from build123d import *

# Parameters (mm, degrees)
SKETCH_1_W      = 3
SKETCH_1_H      = 20
SKETCH_1_W_2    = 20
SKETCH_1_H_2    = 3
EXTRUDE_1_DEPTH = 6
FILLET_2_R      = 15
FILLET_3_R      = 15
FILLET_4_R      = 15
FILLET_5_R      = 15
FILLET_6_R      = 15
FILLET_7_R      = 15
FILLET_8_R      = 15
FILLET_9_R      = 15
FILLET_10_R     = 15
FILLET_11_R     = 15
FILLET_12_R     = 15
FILLET_13_R     = 15
FILLET_14_R     = 15
FILLET_15_R     = 15


with BuildPart() as part:
    # Эскиз1 → Бобышка-Вытянуть1 (new body)
    with BuildSketch(Plane.XY):
        Polygon((118, 244), (118, 129), (268, 129), (268, 244), (293, 244), (293, 250), (313, 250), (313, 244), (356, 244), (356, 250), (376, 250), (376, 244), (386, 244), (386, 147), (392, 147), (392, 97), (386, 97), (386, 0), (366, 0), (366, -6), (346, -6), (346, 0), (203, 0), (203, -6), (183, -6), (183, 0), (40, 0), (40, -6), (20, -6), (20, 0), (0, 0), (0, 97), (-6, 97), (-6, 147), (0, 147), (0, 244), (10, 244), (10, 250), (30, 250), (30, 244), (73, 244), (73, 250), (93, 250), (93, 244), align=None)
        Polygon((20, 20), (20, 224), (88, 224), (88, 99), (183, 99), (183, 20), align=None, mode=Mode.SUBTRACT)
        Polygon((298, 99), (298, 224), (366, 224), (366, 20), (203, 20), (203, 99), align=None, mode=Mode.SUBTRACT)
        with Locations((99.5, 214)):
            Rectangle(SKETCH_1_W, SKETCH_1_H, mode=Mode.SUBTRACT)
        with Locations((99.5, 159)):
            Rectangle(SKETCH_1_W, SKETCH_1_H, mode=Mode.SUBTRACT)
        with Locations((148, 110.5)):
            Rectangle(SKETCH_1_W_2, SKETCH_1_H_2, mode=Mode.SUBTRACT)
        with Locations((238, 110.5)):
            Rectangle(SKETCH_1_W_2, SKETCH_1_H_2, mode=Mode.SUBTRACT)
        with Locations((286.5, 214)):
            Rectangle(SKETCH_1_W, SKETCH_1_H, mode=Mode.SUBTRACT)
        with Locations((286.5, 159)):
            Rectangle(SKETCH_1_W, SKETCH_1_H, mode=Mode.SUBTRACT)
    extrude(amount=EXTRUDE_1_DEPTH)

    # Скругление2
    fillet_2_edges = [part.edges().sort_by_distance(p)[0] for p in [
        (366, 20, 3),
    ]]
    fillet(fillet_2_edges, radius=FILLET_2_R)

    # Скругление3
    fillet_3_edges = [part.edges().sort_by_distance(p)[0] for p in [
        (203, 99, 3),
    ]]
    fillet(fillet_3_edges, radius=FILLET_3_R)

    # Скругление4
    fillet_4_edges = [part.edges().sort_by_distance(p)[0] for p in [
        (203, 20, 3),
    ]]
    fillet(fillet_4_edges, radius=FILLET_4_R)

    # Скругление5
    fillet_5_edges = [part.edges().sort_by_distance(p)[0] for p in [
        (298, 99, 3),
    ]]
    fillet(fillet_5_edges, radius=FILLET_5_R)

    # Скругление6
    fillet_6_edges = [part.edges().sort_by_distance(p)[0] for p in [
        (298, 224, 3),
    ]]
    fillet(fillet_6_edges, radius=FILLET_6_R)

    # Скругление7
    fillet_7_edges = [part.edges().sort_by_distance(p)[0] for p in [
        (366, 224, 3),
    ]]
    fillet(fillet_7_edges, radius=FILLET_7_R)

    # Скругление8
    fillet_8_edges = [part.edges().sort_by_distance(p)[0] for p in [
        (183, 99, 3),
    ]]
    fillet(fillet_8_edges, radius=FILLET_8_R)

    # Скругление9
    fillet_9_edges = [part.edges().sort_by_distance(p)[0] for p in [
        (20, 224, 3),
    ]]
    fillet(fillet_9_edges, radius=FILLET_9_R)

    # Скругление10
    fillet_10_edges = [part.edges().sort_by_distance(p)[0] for p in [
        (88, 99, 3),
    ]]
    fillet(fillet_10_edges, radius=FILLET_10_R)

    # Скругление11
    fillet_11_edges = [part.edges().sort_by_distance(p)[0] for p in [
        (88, 224, 3),
    ]]
    fillet(fillet_11_edges, radius=FILLET_11_R)

    # Скругление12
    fillet_12_edges = [part.edges().sort_by_distance(p)[0] for p in [
        (183, 20, 3),
    ]]
    fillet(fillet_12_edges, radius=FILLET_12_R)

    # Скругление13
    fillet_13_edges = [part.edges().sort_by_distance(p)[0] for p in [
        (20, 20, 3),
    ]]
    fillet(fillet_13_edges, radius=FILLET_13_R)

    # Скругление14
    fillet_14_edges = [part.edges().sort_by_distance(p)[0] for p in [
        (268, 129, 3),
    ]]
    fillet(fillet_14_edges, radius=FILLET_14_R)

    # Скругление15
    fillet_15_edges = [part.edges().sort_by_distance(p)[0] for p in [
        (118, 129, 3),
    ]]
    fillet(fillet_15_edges, radius=FILLET_15_R)


solid = part.part
For this review, take the finished solid that the model builds, in its own axes (mm). A direction names the side the tool comes from. Round coordinates to 2 decimals unless told otherwise and drop trailing zeros. Order: outer loops, then holes, each group sorted by start corner. A loop starts at its lowest first (then second) coordinate and runs counter-clockwise, first axis right, second up. Notation, with made-up numbers: M 86.25,-11 L 107.25,-11 A16 cw 107.25,9 Z; hole C 9.5,28.25 d1. An arc over 180 degrees is marked long. Write each question's results on one line, items separated by ' | '. Start each with the question number.
1. Add section B-B (x = 142.5). State the section outline as (y, z) points, then the cut area to 3 significant figures.
2. To check wall thickness, follow L1, parallel to X at y = 41, z = 0.9; L2, parallel to Y at x = 247, z = 1.15; L3, parallel to X at y = 117, z = 4.3. State the ranges of each line that lie inside material, in increasing order. Write a range as [from, to].
3. Add section C-C (y = 193.5). State the section outline as (x, z) points.
4. Clearance check with flat-ended pins moving along their axes: pin 1 Ø5 at (x, y) = (102.5, 143.5) entering from -Z; pin 2 Ø3 at (y, z) = (248, 3.5) entering from -X; pin 3 Ø2.5 at (x, z) = (100, 2) entering from +Y; pin 4 Ø1.5 at (x, z) = (149, 2) entering from -Y. State where each tip first meets the part, or that it passes through.
5. Add section D-D (x = 309). State the section outline as (y, z) points.
6. Draft analysis for pull direction Y (two halves, no side actions). For faces 4 (the face through (122.51, 133.28, 3.04)), 5 (the face through (196, 124, 0)), 6 (the face through (361.72, 24.51, 3.04)), state which applies: pulls with the +Y half, pulls with the -Y half, needs draft (parallel to the pull), parting line crosses it, or undercut.
7. Tool access review of faces 1 (the face through (263.49, 133.28, 3.04)), 2 (the face through (196, 124, 6)), 3 (the face through (92.28, 103.51, 3.04)): name each direction out of +Z, -Z, +X, -X, +Y, -Y from which nothing blocks a thin tool from reaching the whole face with its end or side.
8. Add section A-A (y = 48). State the section outline as (x, z) points.
Output values:
1) outline: M 0,0 L 20,0 L 20,6 L 0,6 Z; M 99,0 L 109,0 L 109,6 L 99,6 Z; M 112,0 L 129,0 L 129,6 L 112,6 Z | area: 282 mm^2
2) L1: [0, 20], [183, 203], [366, 386] | L2: [0, 20], [99, 109], [112, 129] | L3: [-6, 20], [88, 298], [366, 392]
3) outline: M 0,0 L 20,0 L 20,6 L 0,6 Z; M 88,0 L 118,0 L 118,6 L 88,6 Z; M 268,0 L 298,0 L 298,6 L 268,6 Z; M 366,0 L 386,0 L 386,6 L 366,6 Z
4) pin 1: z = 0 | pin 2: x = 10 | pin 3: y = 244 | pin 4: y = 0
5) outline: M 0,0 L 20,0 L 20,6 L 0,6 Z; M 223.46,0 L 250,0 L 250,6 L 223.46,6 Z
6) face 4: pulls with the +Y half | face 5: needs draft | face 6: undercut
7) face 1: +Z, -Z, +Y | face 2: +Z, +X, -X, +Y, -Y | face 3: +Z, -Z
8) outline: M 0,0 L 20,0 L 20,6 L 0,6 Z; M 183,0 L 203,0 L 203,6 L 183,6 Z; M 366,0 L 386,0 L 386,6 L 366,6 Z
